```python
from build123d import *

# Parameters (mm, degrees)
SKETCH1_R                    = 1.5
BASE_FLANGE1_DEPTH           = 2
EDGE_FLANGE1_STRIP_W         = 9.5
EDGE_FLANGE1_STRIP_H         = 2
EDGE_FLANGE1_STRIP_CUT_DEPTH = 20
EDGE_FLANGE1_DEPTH           = 20
SKETCH9_R                    = 0.75
CUT_EXTRUDE1_DEPTH           = 10
FILLET1_R                    = 3
SCALE1_SCALE                 = 1.8


# Sheet-metal steps are written as plain solids
with BuildPart() as part:
    # Sketch1 → Base-Flange1 (new body)
    with BuildSketch(Plane(origin=(0, 0, 0), x_dir=(1, 0, 0), z_dir=(0, 1, 0))):
        with BuildLine():
            Line((0, 7), (0, -7))
            ThreePointArc((0, -7), (0.878679656, -9.121320344), (3, -10))
            Line((3, -10), (12, -10))
            Line((12, -10), (12, 10))
            Line((12, 10), (3, 10))
            ThreePointArc((3, 10), (0.878679656, 9.121320344), (0, 7))
        make_face()
        with Locations(Location((2.72, 6, 0), (0, 0, 270))):
            Circle(SKETCH1_R, mode=Mode.SUBTRACT)
        with Locations(Location((2.72, -6, 0), (0, 0, 270))):
            Circle(SKETCH1_R, mode=Mode.SUBTRACT)
    extrude(amount=BASE_FLANGE1_DEPTH)

    # Edge-Flange1 strip (across the edge) → Edge-Flange1 strip cut (cut)
    with BuildSketch(Plane(origin=(12, 2, 10), x_dir=(-1, 0, 0), z_dir=(0, 0, -1))):
        with Locations((-2, -1)):
            Rectangle(EDGE_FLANGE1_STRIP_W, EDGE_FLANGE1_STRIP_H)
    extrude(amount=EDGE_FLANGE1_STRIP_CUT_DEPTH, mode=Mode.SUBTRACT)

    # Edge-Flange1 section (across the edge) → Edge-Flange1 (add)
    with BuildSketch(Plane(origin=(12, 2, 10), x_dir=(-1, 0, 0), z_dir=(0, 0, -1))):
        with BuildLine():
            Line((0, 0.75), (0, 6))
            Line((0, 6), (2, 6))
            Line((2, 6), (2, 0.75))
            ThreePointArc((2, 0.75), (2.219669914, 0.219669914), (2.75, 0))
            Line((2.75, 0), (2.75, -2))
            ThreePointArc((2.75, -2), (0.805456352, -1.194543648), (0, 0.75))
        make_face()
    extrude(amount=EDGE_FLANGE1_DEPTH)

    # Sketch9 → Cut-Extrude1 (cut)
    with BuildSketch(Plane.ZY.offset(-10)):
        with Locations(Location((0, 6, 0), (0, 0, 270))):
            Circle(SKETCH9_R)
    extrude(amount=-CUT_EXTRUDE1_DEPTH, mode=Mode.SUBTRACT)

    # Fillet1
    fillet1_edges = [part.edges().sort_by_distance(p)[0] for p in [
        (11, 8, 10),
        (11, 8, -10),
    ]]
    fillet(fillet1_edges, radius=FILLET1_R)


with BuildPart() as part_1:
    # Scale1: scaled about (7.730300008, 2.413989503, 0)
    add(part.part.scale(SCALE1_SCALE).moved(Location((-6.184240006, -1.931191602, 0))))


solid = part_1.part
```
Design review of the part built by this model. Coordinates are the model's own, in mm. A direction names the side the tool comes from. Coordinates: 2 decimals unless noted, no trailing zeros. Write each loop counter-clockwise with the first axis right and the second up, starting at its lowest first coordinate (ties: lowest second). Pieces come first, ordered by that corner, then holes. Notation, with made-up numbers: M -31,-13 L 0,-13 A28 cw 0,18 Z; hole C 1.5,49 d1. An arc over 180 degrees is marked long. Answer as a JSON object with one key per item and string values.
Item 1: Wall thickness on probe 1 along Z at (x, y) = (-3, 0.5); probe 2 along Y at (x, z) = (9.75, -3); probe 3 along X at (y, z) = (7.75, 11.5): over which ranges is each line inside the solid? List them lowest first.
Outcome:
{"probe 1": "-17.52 to -12.89, -8.71 to 8.71, 12.89 to 17.52", "probe 2": "-1.93 to 1.67", "probe 3": "11.82 to 15.42"}
Item 2: Insertion check: pin 1 Ø4.5 at (y, z) = (7, 8.5) entering from -X; pin 2 Ø2 at (x, z) = (10, -3.5) entering from +Y; pin 3 Ø8 at (y, z) = (5, 14.5) entering from -X; pin 4 Ø6 at (x, z) = (-1.29, 10.8) entering from +Y. Each pin has a flat end and moves straight along its axis. Give the tip position at first contact, or say it passes through.
Outcome:
{"pin 1": "x = 11.82", "pin 2": "y = 1.78", "pin 3": "x = -6.18", "pin 4": "y = 1.67"}
Item 3: Add section B-B, the plane y = 9.25. Give the boundary of the cut face in (x, z), and give its area (3 significant figures).
Outcome:
{"outline": "M 11.82,-17.54 L 15.42,-17.54 L 15.42,-1.3 L 11.82,-1.3 Z; M 11.82,1.3 L 15.42,1.3 L 15.42,17.54 L 11.82,17.54 Z", "area": "117 mm²"}
Item 4: Add section C-C, the plane x = 12.75. Give the boundary of the cut face in (y, z), and give its area (3 significant figures).
Outcome:
{"outline": "M -1.37,-18 L 7.07,-18 A5.4 ccw 12.47,-12.6 L 12.47,12.6 A5.4 ccw 7.07,18 L -1.37,18 Z; hole C 8.87,0 d2.7", "area": "480 mm²"}
Item 5: Machinability: for faces 4 (the cylindrical face through (13.591, 10.845, -16.46)), 5 (the flat face through (2, 1.669, 0)), which of the approach directions +Z, -Z, +X, -X, +Y, -Y give a long, thin tool a straight path to every point of the face, cutting with its end or side? Answer none if there is none.
Outcome:
{"face 4": "-Z, +X, -X, +Y", "face 5": "+Z, -Z, -X, +Y"}
Item 6: Add section D-D, the plane y = -0.5. Give the boundary of the cut face in (x, z).
Outcome:
{"outline": "M -6.18,-12.6 A5.4 ccw -0.78,-18 L 13.95,-18 L 13.95,18 L -0.78,18 A5.4 ccw -6.18,12.6 Z; hole C -1.29,-10.8 d5.4; hole C -1.29,10.8 d5.4"}
Item 7: Draft analysis for pull direction Z (two halves, no side actions). For faces 1 (the cylindrical face through (-3.924, -0.156, -11.385)), 2 (the cylindrical face through (13.591, 10.845, 16.46)), 3 (the cylindrical face through (11.431, 2.075, 0.252)), state which applies: pulls with the +Z half, pulls with the -Z half, needs draft (parallel to the pull), parting line crosses it, or undercut.
Outcome:
{"face 1": "undercut", "face 2": "pulls with the +Z half", "face 3": "needs draft"}
Item 8: Add section A-A, the plane z = 0. Give the boundary of the cut face in (x, y).
Outcome:
{"outline": "M -6.18,-1.93 L 10.47,-1.93 A4.95 ccw 15.42,3.02 L 15.42,7.52 L 11.82,7.52 L 11.82,3.02 A1.35 cw 10.47,1.67 L -6.18,1.67 Z; M 11.82,10.22 L 15.42,10.22 L 15.42,12.47 L 11.82,12.47 Z"}
